```python
from build123d import *

# Parameters (mm, degrees)
BOSS_EXTRUDE1_DEPTH = 38.1
CUT_EXTRUDE1_REACH  = 44.121


with BuildPart() as part:
    # Sketch1 → Boss-Extrude1 (new, symmetric)
    with BuildSketch(Plane.XY):
        Polygon((-12.7, 7.62), (-6.35, 7.62), (-6.35, 1.27), (6.35, 1.27), (6.35, 7.62), (12.7, 7.62), (12.7, -7.62), (9.652, -7.62), (9.652, -2.286), (-9.652, -2.286), (-9.652, -11.43), (-12.7, -11.43), align=None)
    extrude(amount=BOSS_EXTRUDE1_DEPTH, both=True)

    # Sketch2 → Cut-Extrude1 (cut, up to next)
    with BuildSketch(Plane(origin=(0, 1.27, 0), x_dir=(1, 0, 0), z_dir=(0, 1, 0)), mode=Mode.PRIVATE) as cut_extrude1_sk1:
        with BuildLine():
            Line((4.191, 2.159), (4.191, -2.159))
            ThreePointArc((4.191, -2.159), (0, -6.35), (-4.191, -2.159))
            Line((-4.191, -2.159), (-4.191, 2.159))
            ThreePointArc((-4.191, 2.159), (0, 6.35), (4.191, 2.159))
        make_face()
    cut_extrude1_tool1 = extrude(cut_extrude1_sk1.sketch, amount=-CUT_EXTRUDE1_REACH, mode=Mode.PRIVATE) & part.part
    add(cut_extrude1_tool1.solids().sort_by_distance((0, 1.27, 0))[0], mode=Mode.SUBTRACT)


solid = part.part
```
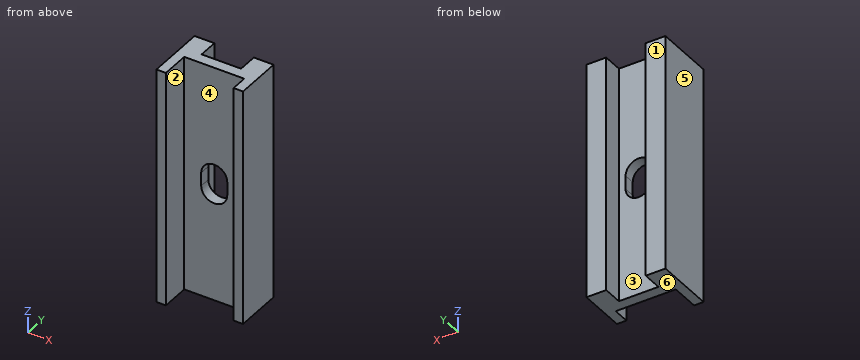
Geometry check sheet. Reference: the model listing, model coordinates, mm. Face numbers are marked on the shaded views. A direction names the side the tool comes from. Give positions to 0.01 mm unless a question says otherwise; leave off trailing zeros. Order: outer loops, then holes, each group sorted by start corner. A loop starts at its lowest first (then second) coordinate and runs counter-clockwise, first axis right, second up.
1. Thickness scan on L1, parallel to X at y = -4.25, z = 2; L2, parallel to X at y = 6.75, z = 30; L3, parallel to Y at x = 10, z = 34.5. Record the ranges inside material, lowest first.
2. Section check B-B, the plane y = -3.25. Enter the section's corners in (x, z).
3. Section check D-D, the plane y = -0.25. Enter the section's corners in (x, z), and give its area (3 significant figures).
4. Release check for a two-part mould opening along X. For the marked faces 3, 4, 5 and 6 record: pulls with the +X half, pulls with the -X half, needs draft (parallel to the pull), parting line crosses it, or undercut.
5. Access from +Z, -Z, +X, -X, +Y, -Y to the whole of each face (thin tool, end or side, straight path). Record for the marked faces 1 and 2.
6. Gauge pin test, flat end, axial feed: pin 1 Ø4 at (x, z) = (9.5, 19) entering from -Y. Record the tip position at first contact, or that the pin passes through.
7. Section check C-C, the plane z = -5. Enter the section's corners in (x, y).
8. Section check A-A, the plane x = 0. Enter the section's corners in (y, z), and give its area (3 significant figures).
Values follow:
1. L1: x = -12.7 to -9.65, 9.65 to 12.7
1. L2: x = -12.7 to -6.35, 6.35 to 12.7
1. L3: y = -7.62 to 7.62
2. outline: (-12.7, -38.1) - (-9.65, -38.1) - (-9.65, 38.1) - (-12.7, 38.1) - close; (9.65, -38.1) - (12.7, -38.1) - (12.7, 38.1) - (9.65, 38.1) - close
3. outline: (-12.7, -38.1) - (12.7, -38.1) - (12.7, 38.1) - (-12.7, 38.1) - close; hole (-4.19, -2.16) arc R4.19 ccw to (4.19, -2.16) - (4.19, 2.16) arc R4.19 ccw to (-4.19, 2.16) - close
3. area: 1,840 mm2
4. face 3: undercut
4. face 4: undercut
4. face 5: pulls with the -X half
4. face 6: needs draft
5. face 1: +Z, -Z, +X, -X, +Y
5. face 2: +Z, -Z, -Y
6. pin 1: stops at y = -7.62
7. outline: (-12.7, -11.43) - (-9.65, -11.43) - (-9.65, -2.29) - (-3.08, -2.29) - (-3.08, 1.27) - (-6.35, 1.27) - (-6.35, 7.62) - (-12.7, 7.62) - close; (3.08, -2.29) - (9.65, -2.29) - (9.65, -7.62) - (12.7, -7.62) - (12.7, 7.62) - (6.35, 7.62) - (6.35, 1.27) - (3.08, 1.27) - close
8. outline: (-2.29, -38.1) - (1.27, -38.1) - (1.27, -6.35) - (-2.29, -6.35) - close; (-2.29, 6.35) - (1.27, 6.35) - (1.27, 38.1) - (-2.29, 38.1) - close
8. area: 226 mm2
